Work out the finished part from the listing and answer in its coordinate system (mm). Face numbers are marked on the shaded views. A direction names the side the tool comes from. Round coordinates to 2 decimals unless told otherwise and drop trailing zeros. Order: outer loops, then holes, each group sorted by start corner. A loop starts at its lowest first (then second) coordinate and runs counter-clockwise, first axis right, second up. Notation, with made-up numbers: M 55.5,12 L 111.5,12 A37 ccw 111.5,48 Z; hole C 66.25,9.5 d7. An arc over 180 degrees is marked long. Answer as a JSON object with one key per item and string values. Group by question number.
from build123d import *

# Parameters (mm, degrees)
SKETCH1_W                 = 3
SKETCH1_H                 = 1.629773482
SKETCH1_H_2               = 1.605700765
BOSS_EXTRUDE21_DEPTH      = 1.5
BOSS_EXTRUDE22_DEPTH      = 0.0001
BOSS_EXTRUDE22_DEPTH_BACK = 5
SKETCH4_W                 = 8
SKETCH4_H                 = 1.27322458
SKETCH5_W                 = 8
SKETCH5_H                 = 1.75
BOSS_EXTRUDE23_DEPTH      = 1.5
SKETCH6_W                 = 3.309716912
SKETCH6_H                 = 3.42211522
SKETCH6_W_2               = 3.309716913
BOSS_EXTRUDE24_DEPTH      = 3
SKETCH8_W                 = 3.309716912
SKETCH8_H                 = 1.8
SKETCH8_W_2               = 3.309716913
BOSS_EXTRUDE26_DEPTH      = 1.5
FILLET1_R                 = 1
FILLET2_R                 = 1
CHAMFER4_SIZE             = 3
FILLET3_R                 = 1.6


with BuildPart() as part:
    # Sketch1 → Boss-Extrude21 (new body)
    # profile 1 of 3: a face of its own
    with BuildSketch(Plane(origin=(0, 0, 0), x_dir=(1, 0, 0), z_dir=(0, 1, 0))):
        with Locations((14.277336143, -0.790814024)):
            Rectangle(SKETCH1_W, SKETCH1_H)
    # profile 2 of 3: a face of its own
    with BuildSketch(Plane(origin=(0, 0, 0), x_dir=(1, 0, 0), z_dir=(0, 1, 0))):
        Polygon((-2.384327038, -10.702702703), (-11.708098218, -10.702702703), (-11.708098218, -9.652730884), (14.939444142, -9.652730884), (14.939444142, -10.702702703), (5.615672962, -10.702702703), (5.615672962, -11.975927283), (21.477336143, -11.975927283), (21.477336143, 0.024072717), (15.777336143, 0.024072717), (15.777336143, -1.605700765), (12.777336143, -1.605700765), (12.777336143, 0.024072717), (-17.922663857, 0.024072717), (-17.922663857, -11.975927283), (-2.384327038, -11.975927283), align=None)
        with Locations((-10.768292904, -0.870035762)):
            Rectangle(SKETCH1_W, SKETCH1_H_2, mode=Mode.SUBTRACT)
    # profile 3 of 3: a face of its own
    with BuildSketch(Plane(origin=(0, 0, 0), x_dir=(1, 0, 0), z_dir=(0, 1, 0))):
        with Locations((-10.768292904, -0.870035762)):
            Rectangle(SKETCH1_W, SKETCH1_H_2)
    extrude(amount=BOSS_EXTRUDE21_DEPTH)

    # Sketch4 → Boss-Extrude22 (add, two sides: drawn at the far end of the back side and taken through both)
    with BuildSketch(Plane.XZ.offset(-BOSS_EXTRUDE22_DEPTH_BACK)):
        with Locations((1.615672962, 11.339314993)):
            Rectangle(SKETCH4_W, SKETCH4_H)
    extrude(amount=BOSS_EXTRUDE22_DEPTH + BOSS_EXTRUDE22_DEPTH_BACK)

    # Sketch5 → Boss-Extrude23 (add)
    with BuildSketch(Plane.XY.offset(11.975927283)):
        with Locations((1.615672962, 4.125)):
            Rectangle(SKETCH5_W, SKETCH5_H)
    extrude(amount=BOSS_EXTRUDE23_DEPTH)

    # Sketch6 → Boss-Extrude24 (add)
    with BuildSketch(Plane(origin=(0, 1.5, 0), x_dir=(1, 0, 0), z_dir=(0, 1, 0))):
        with Locations((14.622477687, -1.686984893)):
            Rectangle(SKETCH6_W, SKETCH6_H)
        with Locations((-11.0678054, -1.686984893)):
            Rectangle(SKETCH6_W_2, SKETCH6_H)
    extrude(amount=BOSS_EXTRUDE24_DEPTH)

    # Sketch8 → Boss-Extrude26 (add)
    with BuildSketch(Plane(origin=(0, 0, -0.024072717), x_dir=(-1, 0, 0), z_dir=(0, 0, -1))):
        with Locations((-14.622477687, 3.6)):
            Rectangle(SKETCH8_W, SKETCH8_H)
        with Locations((11.0678054, 3.6)):
            Rectangle(SKETCH8_W_2, SKETCH8_H)
    extrude(amount=BOSS_EXTRUDE26_DEPTH)

    # Fillet1
    fillet1_edges = [part.edges().sort_by_distance(p)[0] for p in [
        (-11.0678054, 4.5, -1.524072717),
        (1.615672962, 5, 13.475927283),
        (14.622477687, 4.5, -1.524072717),
    ]]
    fillet(fillet1_edges, radius=FILLET1_R)

    # Fillet2
    fillet2_edges = [part.edges().sort_by_distance(p)[0] for p in [
        (21.477336143, 0.75, 11.975927283),
        (-17.922663857, 0.75, 11.975927283),
        (-17.922663857, 0.75, -0.024072717),
        (21.477336143, 0.75, -0.024072717),
    ]]
    fillet(fillet2_edges, radius=FILLET2_R)

    # Chamfer4
    chamfer4_edges = [part.edges().sort_by_distance(p)[0] for p in [
        (14.622477687, 4.5, 3.398042503),
        (-11.0678054, 4.5, 3.398042503),
    ]]
    chamfer(chamfer4_edges, length=CHAMFER4_SIZE - 0.0001)  # a hair under: the kernel refuses the full size

    # Fillet3
    fillet3_edges = [part.edges().sort_by_distance(p)[0] for p in [
        (1.615672962, 5, 10.702702703),
    ]]
    fillet(fillet3_edges, radius=FILLET3_R)


solid = part.part
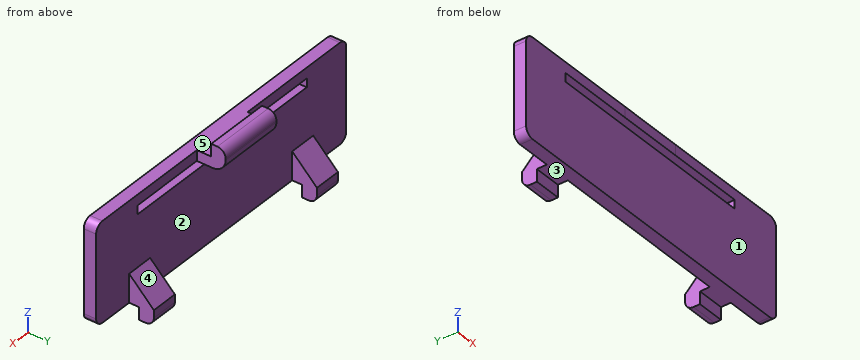
Item 1: Consider L1, parallel to X at y = 4.15, z = -0.5; L2, parallel to Z at x = 1, y = 1; L3, parallel to Y at x = 0, z = 8.75. Determine where each line is inside the solid, lowest interval first.
Item 2: Find section D-D (z = 4.75). Give the vertices of the cut face in (x, y), and give its area (3 significant figures).
Item 3: Find section A-A (x = 4). Give the vertices of the cut face in (y, z), and give its area (3 significant figures).
Item 4: A tool of negligible diameter and unlimited length cuts with its end or side. For the marked faces 3, 4 and 5, from which of +Z, -Z, +X, -X, +Y, -Y can it reach the whole face along a straight path? Write none if from no direction.
Item 5: Find section C-C (z = 2.25). Give the vertices of the cut face in (x, y), and give its area (3 significant figures).
Item 6: Each of these flat-tipped pins is pushed along its axis until it touches: pin 1 (0.5 mm diameter, centred on x = 14, z = 0, fed in from +Y); pin 2 (3 mm diameter, centred on y = 3.5, z = 11.5, fed in from +X); pin 3 (2.5 mm diameter, centred on y = 3.5, z = 2, fed in from +X). Where does it stop, or does it pass through?
Item 7: Find section B-B (y = 0.45). Give the vertices of the cut face in (x, z), and give its area (3 significant figures).
Item 8: The mould has two halves that part along X. Classify the marked faces 1 and 2: +X half, -X half, draft (parallel to the pull), parting line (faces both ways), or undercut.
Responses:
{
 "1": {"L1": "x = -12.72 to -9.41, 12.97 to 16.28", "L2": "z = -0.02 to 9.65, 10.7 to 11.98", "L3": "y = 0 to 1.5"},
 "2": {"outline": "M -17.92,0 L 21.48,0 L 21.48,1.5 L -17.92,1.5 Z", "area": "59.1 mm^2"},
 "3": {"outline": "M 0,-0.02 L 1.5,-0.02 L 1.5,9.65 L 0,9.65 Z; M 0,10.7 L 3.4,10.7 A1.6 ccw 5,12.3 L 5,12.48 A1 ccw 4,13.48 L 3.25,13.48 L 3.25,11.98 L 0,11.98 Z", "area": "22.7 mm^2"},
 "4": {"face 3": "-Z, +X, -X, -Y", "face 4": "+Z, +X, -X, +Y", "face 5": "+Z, +X, -X, -Y"},
 "5": {"outline": "M -17.92,0 L 21.48,0 L 21.48,1.5 L 16.28,1.5 L 16.28,2.65 L 12.97,2.65 L 12.97,1.5 L -9.41,1.5 L -9.41,2.65 L -12.72,2.65 L -12.72,1.5 L -17.92,1.5 Z", "area": "66.7 mm^2"},
 "6": {"pin 1": "stops at y = 4.5", "pin 2": "stops at x = 5.62", "pin 3": "stops at x = 16.28"},
 "7": {"outline": "M -17.92,0.98 A1 ccw -16.92,-0.02 L 20.48,-0.02 A1 ccw 21.48,0.98 L 21.48,10.98 A1 ccw 20.48,11.98 L -16.92,11.98 A1 ccw -17.92,10.98 Z; hole M -11.71,9.65 L 14.94,9.65 L 14.94,10.7 L -11.71,10.7 Z", "area": "444 mm^2"},
 "8": {"face 1": "draft", "face 2": "undercut"}
}
